Verification items for this drawing (mm, ordinates from the low corner). Round coordinates to 2 decimals unless told otherwise and drop trailing zeros. Order: outer loops, then holes, each group sorted by start corner. A loop starts at its lowest first (then second) coordinate and runs counter-clockwise, first axis right, second up. Notation, with made-up numbers: (43.5, 20.5) -> (94.5, 20.5) arc R11 ccw to (94.5, 24.5) -> close; hole circle Ø6 at (61, -6.5). An arc over 180 degrees is marked (long way). Answer in a Markdown table with one row per item. Add a question column.
1. Depth check by flat-ended pin: P1, Ø2, axis at x = 12.5, y = 12, coming from the -Z side; P2, Ø2, axis at x = 10, y = 6.5, coming from the +Z side. Enter the tip coordinate at first touch or a pass-through.
2. Sectioned sample at A-A, the plane y = 8.4. Record the boundary of the cut face in (x, z).
3. Draft check along Z on the marked faces 1, 2 and 3. Enter one of: +Z half, -Z half, draft (parallel to the pull), parting line (faces both ways), or undercut.
4. Material ranges on L1, parallel to Y at x = 9.75, z = 8.4; L2, parallel to Z at x = 6.5, y = 6; L3, parallel to Y at x = 4.5, z = 9.25, recorded low to high. Write a range as from..to.
5. Sectioned sample at B-B, the plane x = 6.75. Record the boundary of the cut face in (y, z).
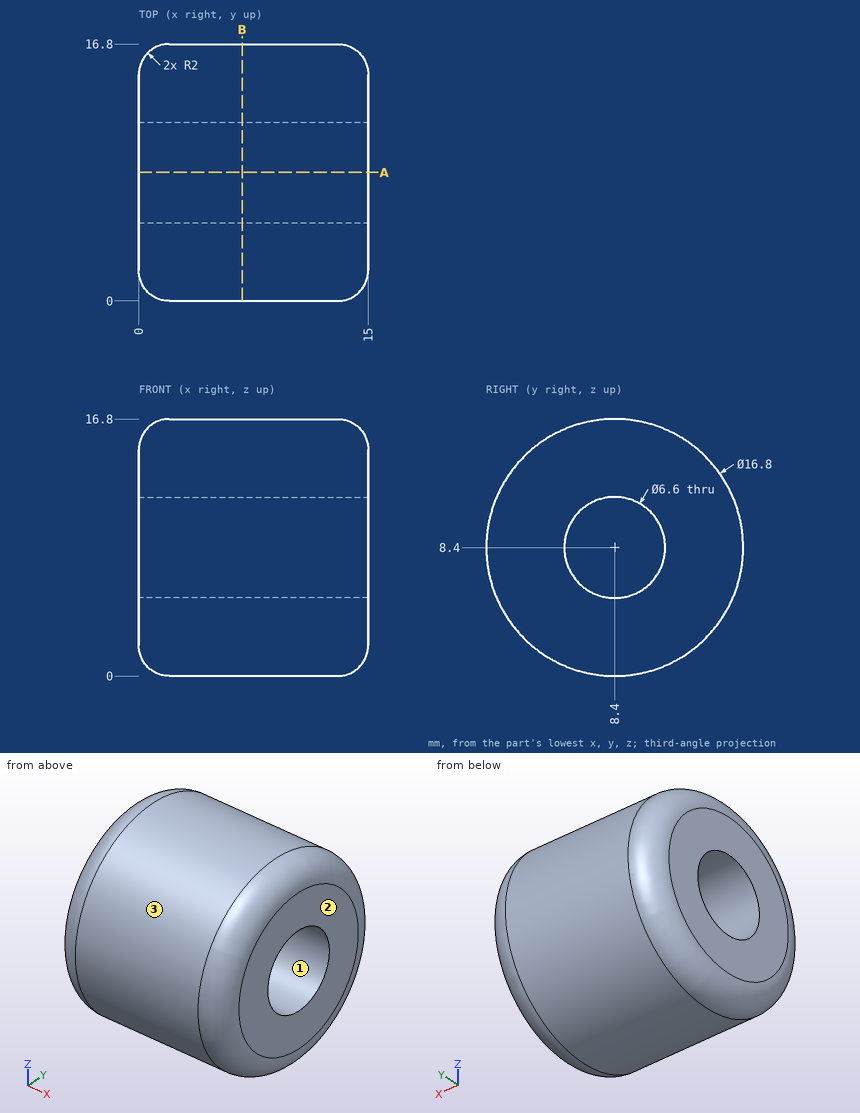
Answer key:
| question | item | result |
|---|---|---|
| 1 | P1 | stops at z = 0.41 |
| 1 | P2 | stops at z = 16.75 |
| 2 | outline | (0, 2) arc R2 ccw to (2, 0) -> (13, 0) arc R2 ccw to (15, 2) -> (15, 5.1) -> (0, 5.1) -> close; (0, 11.7) -> (15, 11.7) -> (15, 14.8) arc R2 ccw to (13, 16.8) -> (2, 16.8) arc R2 ccw to (0, 14.8) -> close |
| 3 | face 1 | undercut |
| 3 | face 2 | draft |
| 3 | face 3 | parting line |
| 4 | L1 | y = 0..5.1, 11.7..16.8 |
| 4 | L2 | z = 0.35..6.14, 10.66..16.45 |
| 4 | L3 | y = 0.04..5.21, 11.59..16.76 |
| 5 | outline | circle Ø16.8 at (8.4, 8.4); hole circle Ø6.6 at (8.4, 8.4) |
